Design review of the part built by this model. Coordinates are the model's own, in mm. Face numbers are marked on the shaded views. A direction names the side the tool comes from. Give positions to 0.01 mm unless a question says otherwise; leave off trailing zeros. Write each loop counter-clockwise with the first axis right and the second up, starting at its lowest first coordinate (ties: lowest second). Pieces come first, ordered by that corner, then holes. Notation, with made-up numbers: (39, 81) - (44, 81) arc R13 ccw to (44, 87) - close; hole circle Ø1 at (11.25, -25.5). An arc over 180 degrees is marked (long way). Write each question's results on one line, items separated by ' | '. Start each with the question number.
from build123d import *

# Parameters (mm, degrees)
F1_DEPTH = 25.4
F2_DEPTH = 50.8


with BuildPart() as f1:
    # F0 (on Top) → F1 (new body)
    with BuildSketch(Plane.XY):
        Polygon((82.166834, 18.702962), (31.366834, -6.697038), (31.366834, -32.097038), (82.166834, -57.497038), align=None)
    extrude(amount=F1_DEPTH)

    # F0 (on Top) → F2 (join)
    with BuildSketch(Plane.XY):
        Polygon((31.366834, 18.702962), (-70.233166, 18.702962), (-70.233166, -57.497038), (31.366834, -57.497038), (31.366834, -32.097038), (31.366834, -6.697038), align=None)
        Polygon((82.166834, 18.702962), (31.366834, -6.697038), (31.366834, -32.097038), (82.166834, -57.497038), align=None)
    extrude(amount=F2_DEPTH)


solid = f1.part
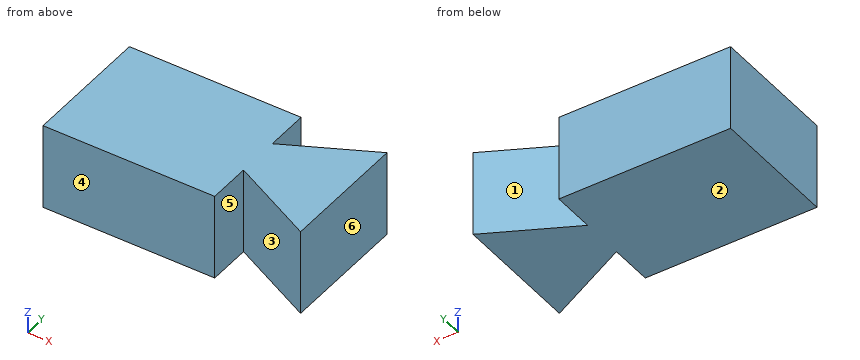
Q1. The part is to be moulded in two halves that separate along X. For the marked faces 4, 5 and 6, say which applies: +X half, -X half, draft (parallel to the pull), parting line (faces both ways), or undercut.
Q2. Add section B-B on z = 35. State the section outline as (x, y) points.
Q3. Add section D-D on x = 66. State the section outline as (y, z) points.
Q4. Add section A-A on y = -50.5. State the section outline as (x, z) points.
Q5. Machinability: for the marked faces 1, 2 and 3, which of the approach directions +Z, -Z, +X, -X, +Y, -Y give a long, thin tool a straight path to every point of the face, cutting with its end or side? Answer none if there is none.
Q6. Insertion check: P1, Ø10, axis at x = 42.5, z = 13, coming from the +Y side; P2, Ø1.5, axis at x = 46.5, z = 23.5, coming from the +Y side. Each pin has a flat end and moves straight along its axis. Give the tip position at first contact, or say it passes through.
Q7. Add section C-C on y = 0.5. State the section outline as (x, z) points, plus the area to 3 significant figures.
Q8. For line 1 along X through (y, z) = (5, 39.5); line 2 along X through (y, z) = (-44, 39), list the stretches that pass through material, from the lowest coordinate up. Write a range as [from, to].
Result:
1) face 4: draft | face 5: undercut | face 6: +X half
2) outline: (-70.23, -57.5) - (31.37, -57.5) - (31.37, -32.1) - (82.17, -57.5) - (82.17, 18.7) - (31.37, -6.7) - (31.37, 18.7) - (-70.23, 18.7) - close
3) outline: (-49.41, 0) - (10.62, 0) - (10.62, 50.8) - (-49.41, 50.8) - close
4) outline: (-70.23, 0) - (31.37, 0) - (31.37, 50.8) - (-70.23, 50.8) - close; (68.17, 0) - (82.17, 0) - (82.17, 50.8) - (68.17, 50.8) - close
5) face 1: +Z, -Z, +Y | face 2: -Z, +X, -X, +Y, -Y | face 3: +Z, -Z, -Y
6) P1: stops at y = 1.37 | P2: stops at y = 1.24
7) outline: (-70.23, 0) - (31.37, 0) - (31.37, 50.8) - (-70.23, 50.8) - close; (45.76, 0) - (82.17, 0) - (82.17, 50.8) - (45.76, 50.8) - close | area: 7,010 mm²
8) line 1: x = [-70.23, 31.37], [54.76, 82.17] | line 2: x = [-70.23, 31.37], [55.17, 82.17]
